Input: dimensioned drawing with shaded views. Units: mm. Origin: part minimum x, y, z. A direction names the side the tool comes from. Round coordinates to 2 decimals unless told otherwise and drop trailing zeros. Order: outer loops, then holes, each group sorted by start corner. A loop starts at its lowest first (then second) coordinate and runs counter-clockwise, first axis right, second up. Notation, with made-up numbers: M 74,13.5 L 107,13.5 A19 cw 107,21.5 Z; hole C 73.5,84 d11. An arc over 180 degrees is marked long. Answer as CSV lines item,"result". Start each with the question number.
Item 1: Section query A-A on y = 7.5. Return the cut outline in (x, z), plus the area to 3 significant figures.
Item 2: Line query: line 1 (X direction, y = 10.9, z = 10); line 2 (X direction, y = 2.25, z = 6.75); line 3 (Y direction, x = 42.5, z = 18.75). Output: solid intervals per line, ascending. Write a range as [from, to].
Item 3: First-contact query: P1, Ø3, axis at x = 37, z = 13.5, coming from the +Y side; P2, Ø5, axis at x = 35, z = 10, coming from the -Y side; P3, Ø11, axis at y = 7, z = 9.5, coming from the -X side. Flat tips, straight axial feed; report the tip coordinate or a pass-through.
Item 4: Set-up query: the marked faces 5, 6 and 7. Return all of +Z, -Z, +X, -X, +Y, -Y with unobstructed straight access to the full face (end or side cutting, diameter ignored); none if empty.
Item 5: Section query B-B on z = 10. Return the cut outline in (x, y), plus the area to 4 significant figures.
Item 6: Pull-direction query (X, two-part tool) for the marked faces 1, 2, 3 and 4; classes: +X half, -X half, draft (parallel to the pull), parting line (faces both ways), or undercut.
Item 7: Section query C-C on x = 15. Return the cut outline in (y, z), plus the area to 4 significant figures.
Item 8: Section query D-D on y = 11.75. Return the cut outline in (x, z), plus the area to 3 significant figures.
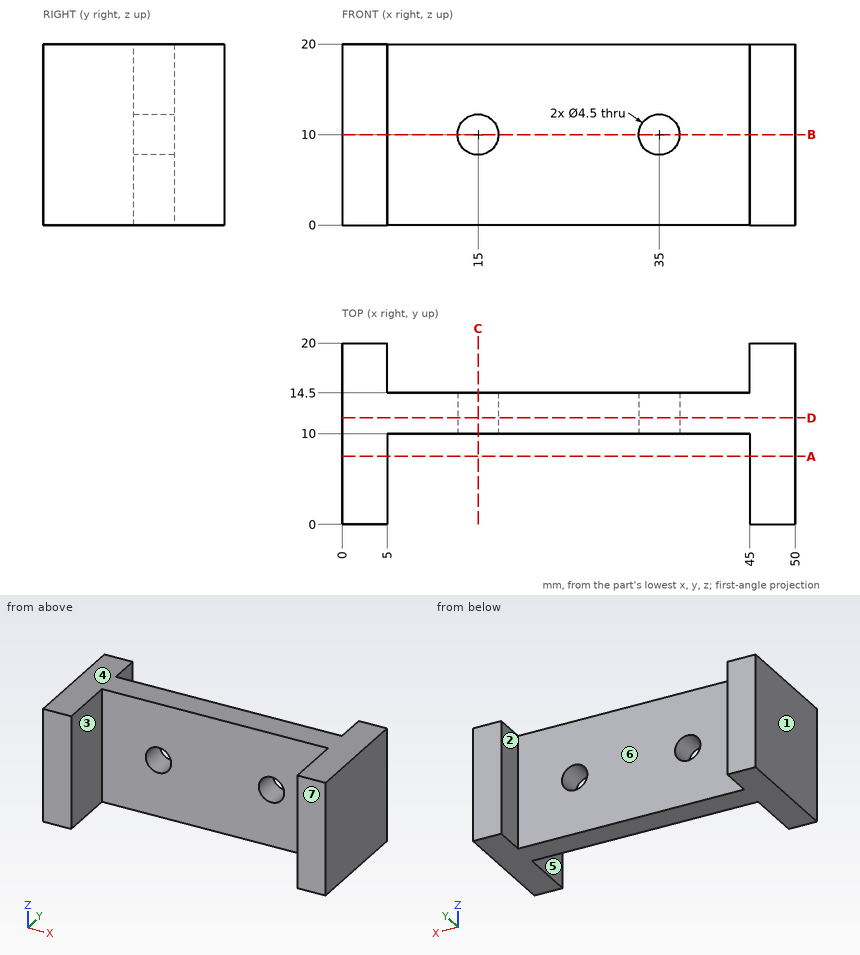
Results:
1,outline,"M 0,0 L 5,0 L 5,20 L 0,20 Z; M 45,0 L 50,0 L 50,20 L 45,20 Z"
1,area,"200 mm^2"
2,line 1,"[0, 12.75], [17.25, 32.75], [37.25, 50]"
2,line 2,"[0, 5], [45, 50]"
2,line 3,"[10, 14.5]"
3,P1,"y = 14.5"
3,P2,"y = 10"
3,P3,"x = 0"
4,face 5,"+Z, -Z, -Y"
4,face 6,"+Z, -Z, +Y"
4,face 7,"+Z, -Z, +X, -X, -Y"
5,outline,"M 0,0 L 5,0 L 5,10 L 12.75,10 L 12.75,14.5 L 5,14.5 L 5,20 L 0,20 Z; M 17.25,10 L 32.75,10 L 32.75,14.5 L 17.25,14.5 Z; M 37.25,10 L 45,10 L 45,0 L 50,0 L 50,20 L 45,20 L 45,14.5 L 37.25,14.5 Z"
5,area,"339.5 mm^2"
6,face 1,"-X half"
6,face 2,"undercut"
6,face 3,"undercut"
6,face 4,"draft"
7,outline,"M 10,0 L 14.5,0 L 14.5,7.75 L 10,7.75 Z; M 10,12.25 L 14.5,12.25 L 14.5,20 L 10,20 Z"
7,area,"69.75 mm^2"
8,outline,"M 0,0 L 50,0 L 50,20 L 0,20 Z; hole C 15,10 d4.5; hole C 35,10 d4.5"
8,area,"968 mm^2"
